Work out the finished part from the listing and answer in its coordinate system (mm). Face numbers are marked on the shaded views. A direction names the side the tool comes from. Give positions to 0.01 mm unless a question says otherwise; leave off trailing zeros. Write each loop counter-clockwise with the first axis right and the second up, starting at its lowest first coordinate (ties: lowest second). Pieces come first, ordered by that corner, then holes. Notation, with made-up numbers: (18, 42.5) - (63, 42.5) arc R30 cw to (63, 72.5) - close; hole circle Ø8 at (52.5, 73.25). An arc over 180 degrees is marked (long way). Write item = value, one per line.
Autodesk Fusion 360 part; units mm, degrees
sketch "Sketch1" plane through (0, 0, 0) normal (1, 0, 0) x (0, 0, -1)
  line L0 (0, 0) -> (0, 45)
  line L1 (0, 0) -> (0, -45)
  line L2 (0, 45) -> (37.5, 45)
  line L3 (0, 45) -> (-37.5, 45)
  line L4 (0, -45) -> (37.5, -45)
  line L5 (0, -45) -> (-37.5, -45)
  arc A0 (-37.5, 45) -> (-37.5, -45) centre (79.119, 0) ccw
  arc A1 (37.5, -45) -> (37.5, 45) centre (-79.119, 0) ccw
  dimension "d1" = 45
  dimension "d2" = 45
  dimension "d3" = 37.5
  dimension "d4" = 37.5
  dimension "d5" = 37.5
  dimension "d6" = 37.5
  dimension "d8" = 125
extrude "Extrude1" add sketch "Sketch1" along normal blind 100
extrude "Extrude2" add 1 faces at (100, -15.2642, -14.2806) along direction (1, 0, 0) blind 35 draft -15
sketch "Sketch2" plane through (135, 0, 0) normal (1, 0, 0) x (0, 0, -1)
  line L0 (-30.8786, -35.6218) -> (30.8786, -35.6218)
  arc A0 (30.8786, -35.6218) -> (30.8786, 35.6218) centre (-79.119, 0) ccw
  line L1 (30.8786, 35.6218) -> (-30.8786, 35.6218)
  arc A1 (-30.8786, 35.6218) -> (-30.8786, -35.6218) centre (79.119, 0) ccw
  circle A2 centre (0, 0) radius 34.5
  dimension "d13" = 69
extrude "Extrude3" add sketch "Sketch2" along normal blind 10 contours A2
sketch "Sketch3" plane through (145, 0, 0) normal (1, 0, 0) x (0, 0, -1)
  circle A0 centre (0, 0) radius 34.5
  circle A1 centre (0, 0) radius 31
  dimension "d16" = 62
extrude "Extrude4" add sketch "Sketch3" along normal blind 30 contours A1
sketch "Sketch4" plane through (175, 0, 0) normal (1, 0, 0) x (0, 0, -1)
  circle A0 centre (0, 0) radius 31
  line L0 (0, 0) -> (27, 0)
  circle A1 centre (27, 0) radius 2.5
  circle A2 centre (27, 0) radius 1.5
  dimension "d19" = 27
  dimension "d20" = 5
  dimension "d21" = -1
extrude "Extrude5" add sketch "Sketch4" along normal blind 1 contours A1
pattern_circular "C-Pattern1" count 12 over 360 about axis through (175, 0, 0) along (1, 0, 0) of "Extrude5"
sketch "Sketch5" plane through (175, 0, 0) normal (1, 0, 0) x (0, 0, -1)
  circle A0 centre (27, 0) radius 2.5
  circle A1 centre (0, 0) radius 31
  circle A2 centre (23.3827, 13.5) radius 2.5
  circle A3 centre (13.5, 23.3827) radius 2.5
  circle A4 centre (0, 27) radius 2.5
  circle A5 centre (-13.5, 23.3827) radius 2.5
  circle A6 centre (-23.3827, 13.5) radius 2.5
  circle A7 centre (-27, 0) radius 2.5
  circle A8 centre (-23.3827, -13.5) radius 2.5
  circle A9 centre (-13.5, -23.3827) radius 2.5
  circle A10 centre (0, -27) radius 2.5
  circle A11 centre (13.5, -23.3827) radius 2.5
  circle A12 centre (23.3827, -13.5) radius 2.5
  line L0 (0, 0) -> (16, 0)
  line L1 (16, 0) -> (16, 17)
  line L2 (16, 0) -> (16, -17)
  line L3 (0, 0) -> (0, -8.0593)
  line L4 (-16, 0) -> (-16, 17)
  line L5 (-16, 0) -> (-16, -17)
  arc A13 (16, 17) -> (-16, 17) centre (0, 1.9003) ccw
  arc A14 (-16, -17) -> (16, -17) centre (0, -1.9003) ccw
  dimension "d26" = 16
  dimension "d27" = 17
  dimension "d28" = 17
  dimension "d29" = 22
extrude "Extrude6" add sketch "Sketch5" along normal blind 100 contours L1 L2 L4 L5 A13 A14
sketch "Sketch6" plane through (275, 0, 0) normal (1, 0, 0) x (0, 0, -1)
  line L0 (-16, 17) -> (-16, -17)
  arc A0 (-16, -17) -> (16, -17) centre (0, -1.9003) ccw
  line L1 (16, -17) -> (16, 17)
  arc A1 (16, 17) -> (-16, 17) centre (0, 1.9003) ccw
  circle A2 centre (0, 0) radius 31
  circle A3 centre (0, 0) radius 30
  dimension "d32" = 62
  dimension "d35" = -1
extrude "Extrude7" add sketch "Sketch6" along normal blind 10 contours L0 A0 L1 A1 | A2 | A3
sketch "Sketch7" plane through (285, 0, 0) normal (1, 0, 0) x (0, 0, -1)
  circle A0 centre (0, 0) radius 31
  circle A1 centre (0, 0) radius 30
  dimension "d36" = -1
extrude "Extrude8" add sketch "Sketch7" along normal blind 1 contours A1
sketch "Sketch8" plane through (286, 0, 0) normal (1, 0, 0) x (0, 0, -1)
  circle A0 centre (0, 0) radius 30
  circle A1 centre (0, 0) radius 31
  dimension "d39" = 62
extrude "Extrude9" add sketch "Sketch8" along normal blind 10 contours A0 | A1
ref_plane "WorkPlane1" through (0, 45, 37.5) normal (0, 0, 1) x (1, 0, 0)
sketch "Sketch9" plane through (0, 0, 37.5) normal (0, 0, 1) x (1, 0, 0)
  circle A0 centre (50, -45) radius 42.5
  dimension "d43" = 85
extrude "Extrude10" add sketch "Sketch9" along normal mid plane 21
sketch "Sketch10" plane through (0, 0, 27) normal (0, 0, -1) x (-1, 0, 0)
  line L0 (-7.5, -45) -> (-92.5, -45)
  arc A0 (-92.5, -45) -> (-7.5, -45) centre (-50, -45) ccw
  line L1 (-50, -45) -> (-50, -75)
  line L2 (-70, -45) -> (-70, -74.9351)
  line L3 (-30, -45) -> (-30, -74.738)
  arc A1 (-70, -74.9351) -> (-30, -74.738) centre (-50.1102, -52.4763) ccw
  dimension "d46" = 30
  dimension "d47" = 20
  dimension "d48" = -20
  dimension "d49" = 30
extrude "Extrude11" add sketch "Sketch10" along normal blind 35 contours L0 L2 L3 A1
sketch "Sketch11" plane through (70, 0, 0) normal (1, 0, 0) x (0, 0, -1)
  line L0 (-27, -45) -> (-27, -74.9351)
  line L1 (-27, -74.9351) -> (8, -74.9351)
  line L2 (8, -74.9351) -> (8, -45)
  line L3 (8, -45) -> (-27, -45)
  line L4 (8, -45) -> (33, -45)
  arc A0 (8, -87) -> (33, -45) centre (-21.8393, -40.7981) ccw
  line L5 (8, -45) -> (8, -87)
  dimension "d52" = 25
  dimension "d54" = 55
extrude "Extrude12" add sketch "Sketch11" against normal blind 40 contours L2 L4 A0 L5
extrude "Extrude13" cut 1 faces at (50.0367, -85.4921, -8) along direction (0, 0, -1) blind 40
sketch "SideDiskHoleSketch" plane through (0, 0, 48) normal (0, 0, 1) x (1, 0, 0)
  circle A0 centre (50, -45) radius 42.5
  circle A1 centre (50, -45) radius 15
extrude "SideDiskHoleCut" cut sketch "SideDiskHoleSketch" against normal blind 20 contours A1
sketch "AxialEndHoleSketch" plane through (296, 0, 0) normal (1, 0, 0) x (0, 0, -1)
  circle A0 centre (0, 0) radius 31
  circle A1 centre (0, 0) radius 15
extrude "AxialEndHoleCut" cut sketch "AxialEndHoleSketch" against normal blind 20 contours A1
equation "d44 = ( 21 / 2 ) * 1 mm"
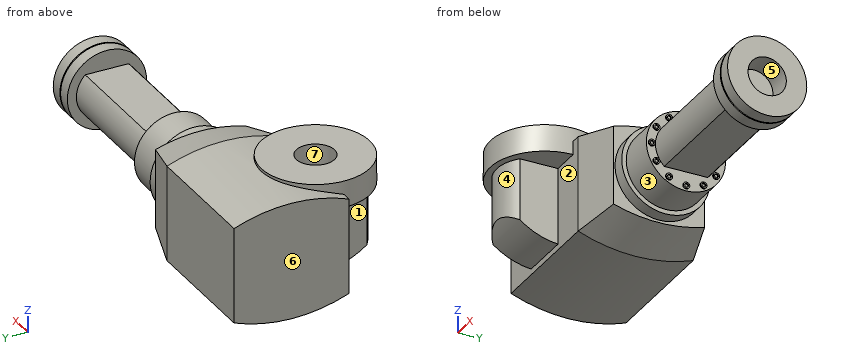
1. Find section B-B, the plane y = -66. Give the vertices of the cut face in (x, z).
Solution:
outline = (13.05, 27) - (30, 27) - (30, -27.05) - (70, -27.05) - (70, 27) - (86.95, 27) - (86.95, 48) - (13.05, 48) - close
2. Given pin 1 (1.5 mm diameter, centred on x = 238, y = 12.5, fed in from +Z); pin 2 (3 mm diameter, centred on x = 223.5, z = 9, fed in from -Y); pin 3 (12 mm diameter, centred on y = -71.5, z = -25.5, fed in from +X), each flat-ended and moving along its own axis, determine where each tip first touches the part or whether it passes through.
Solution:
pin_1 = 16
pin_2 = -22.58
pin_3 = 70
3. For a pull along Y with two mould halves and no side action, classify the marked faces 4, 5, 6 and 7 as pulls with the +Y half, pulls with the -Y half, needs draft (parallel to the pull), parting line crosses it, or undercut.
Solution:
face_4 = pulls with the -Y half
face_5 = undercut
face_6 = needs draft
face_7 = undercut
4. A tool of negligible diameter and unlimited length cuts with its end or side. For the marked faces 1, 2 and 3, from which of +Z, -Z, +X, -X, +Y, -Y can it reach the whole face along a straight path? Write none if from no direction.
Solution:
face_1 = -Z, -X, -Y
face_2 = -Z, -Y
face_3 = +X
5. Find section A-A, the plane x = 73.5. Give the vertices of the cut face in (y, z), then the cut area to 3 significant figures.
Solution:
outline = (-80.41, 27) - (-45, 27) - (-45, -37.5) arc R125 ccw to (45, -37.5) - (45, 37.5) arc R125 ccw to (-9.59, 45.51) - (-9.59, 48) - (-80.41, 48) - close
area = 8,700 mm^2
6. Find section C-C, the plane x = 196. Give the vertices of the cut face in (y, z).
Solution:
outline = (-17, -16) - (17, -16) arc R22 ccw to (17, 16) - (-17, 16) arc R22 ccw to start
7. Straight lines are drawn through the part: line 1 (X direction, y = 25.5, z = -17.5); line 2 (Z direction, x = 175.65, y = 13.5); line 3 (X direction, y = 27, z = 8). For each, find the intervals that lie inside material, in ascending order.
Solution:
line_1 = 0 to 175, 275 to 285, 286 to 296
line_2 = -25.88 to -24.88, -21.88 to -20.88, -16 to 16, 20.88 to 21.88, 24.88 to 25.88
line_3 = 0 to 175, 275 to 296
